The listing builds one solid part. Answer for the finished solid, in the listing's coordinates (mm). Round coordinates to 2 decimals unless told otherwise and drop trailing zeros. Loops run counter-clockwise (first coordinate to the right, second up) from the corner with the lowest first, then second, coordinate; pieces in that order, holes last. Notation, with made-up numbers: (30.25, -2) -> (60.25, -2) arc R12 cw to (60.25, 8) -> close; hole circle Ø6 at (47, -3.75). An arc over 180 degrees is marked (long way). Write each question's results on one line, items separated by ' | '. Start each with the question number.
from build123d import *

# Parameters (mm, degrees)
SM_BASE_FLANGE_1_DEPTH = 3
CUT_EXTRUDE_1_DEPTH    = 10
FILLET_1_R             = 5
FILLET_2_R             = 5
SKETCH_3_R             = 2
CUT_EXTRUDE_2_DEPTH    = 10
SKETCH_5_R             = 2
CUT_EXTRUDE_4_DEPTH    = 10
CHAMFER_1_SIZE         = 1.9
SKETCH_6_R             = 2
CUT_EXTRUDE_5_DEPTH    = 10


# Sheet-metal steps are written as plain solids
with BuildPart() as part:
    # Sketch 1 → Базовая кромка1 (new body)
    with BuildSketch(Plane(origin=(0, 0, 0), x_dir=(1, 0, 0), z_dir=(0, 1, 0))):
        with BuildLine():
            Line((-218.547787293, 260.45511066), (-257.115043875, 306.417777248))
            ThreePointArc((-257.115043875, 306.417777248), (0, 400), (257.115043875, 306.417777248))
            Line((257.115043875, 306.417777248), (218.547787293, 260.45511066))
            ThreePointArc((218.547787293, 260.45511066), (0, 340), (-218.547787293, 260.45511066))
        make_face()
    extrude(amount=-SM_BASE_FLANGE_1_DEPTH)

    # Эскиз2 → Вырез-Вытянуть1 (cut)
    with BuildSketch(Plane(origin=(0, 0, 0), x_dir=(1, 0, 0), z_dir=(0, 1, 0))):
        Polygon((-185.870849123, 267.003439601), (-232.668944094, 335.207852497), (-262.024399195, 311.215696318), (-219.773904278, 254.720487984), align=None)
    extrude(amount=-CUT_EXTRUDE_1_DEPTH, mode=Mode.SUBTRACT)

    # Скругление1
    fillet_1_edges = [part.edges().sort_by_distance(p)[0] for p in [
        (-194.171567718, -1.5, -279.101061069),
        (-228.118354699, -1.5, -328.575738985),
    ]]
    fillet(fillet_1_edges, radius=FILLET_1_R)

    # Скругление2
    fillet_2_edges = [part.edges().sort_by_distance(p)[0] for p in [
        (257.115043875, -1.5, -306.417777248),
        (218.547787293, -1.5, -260.45511066),
    ]]
    fillet(fillet_2_edges, radius=FILLET_2_R)

    # Эскиз3 → Вырез-Вытянуть2 (cut)
    with BuildSketch(Plane(origin=(0, 0, 0), x_dir=(1, 0, 0), z_dir=(0, 1, 0))):
        with Locations(Location((-221.164496487, 327.278574755, 0), (0, 0, 270))):
            Circle(SKETCH_3_R)
        with Locations(Location((-192.875196767, 286.049223862, 0), (0, 0, 270))):
            Circle(SKETCH_3_R)
        with Locations(Location((217.908212497, 267.471514233, 0), (0, 0, 270))):
            Circle(SKETCH_3_R)
        with Locations(Location((250.050541416, 305.777250197, 0), (0, 0, 270))):
            Circle(SKETCH_3_R)
    extrude(amount=-CUT_EXTRUDE_2_DEPTH, mode=Mode.SUBTRACT)

    # Эскиз5 → Вырез-Вытянуть4 (cut)
    with BuildSketch(Plane(origin=(0, 0, 0), x_dir=(1, 0, 0), z_dir=(0, 1, 0))):
        with Locations(Location((15.5203425, 344.65072025, 0), (0, 0, 270))):
            Circle(SKETCH_5_R)
        with Locations(Location((17.7696675, 394.600099996, 0), (0, 0, 270))):
            Circle(SKETCH_5_R)
        with Locations(Location((-106.904799365, 380.258285738, 0), (0, 0, 270))):
            Circle(SKETCH_5_R)
        with Locations(Location((-93.372546281, 332.124325518, 0), (0, 0, 270))):
            Circle(SKETCH_5_R)
    extrude(amount=-CUT_EXTRUDE_4_DEPTH, mode=Mode.SUBTRACT)

    # Фаска1
    chamfer_1_edges = [part.edges().sort_by_distance(p)[0] for p in [
        (-93.372546281, -3, -334.124325518),
        (-221.164496487, -3, -329.278574755),
        (-192.875196767, -3, -288.049223862),
        (217.908212497, -3, -269.471514233),
        (250.050541416, -3, -307.777250197),
        (15.5203425, -3, -346.65072025),
        (17.7696675, -3, -396.600099996),
        (-106.904799365, -3, -382.258285738),
    ]]
    chamfer(chamfer_1_edges, length=CHAMFER_1_SIZE)

    # Эскиз6 → Вырез-Вытянуть5 (cut)
    with BuildSketch(Plane(origin=(0, 0, 0), x_dir=(1, 0, 0), z_dir=(0, 1, 0))):
        with Locations(Location((140.650436017, 369.110355921, 0), (0, 0, 270))):
            Circle(SKETCH_6_R)
        with Locations(Location((122.846583356, 322.387526058, 0), (0, 0, 270))):
            Circle(SKETCH_6_R)
    extrude(amount=-CUT_EXTRUDE_5_DEPTH, mode=Mode.SUBTRACT)


solid = part.part
Item 1: Straight lines are drawn through the part: L1, parallel to X at y = -2.75, z = -296.5; L2, parallel to Z at x = 5.5, y = -0.5; L3, parallel to X at y = -0.65, z = -303. For each, find the intervals that lie inside material, in ascending order. Write a range as [from, to].
Item 2: The part is cut by section C-C, the plane z = -353. Give the vertices of the cut face in (x, y).
Item 3: Determine the mould class of faces 1 (the cylindrical face through (18.4, -1.5, -339.5)), 2 (the flat face through (238.035, -1.479, -283.679)), 3 (the flat face through (18, -3, -363)) for opening direction X: +X half, -X half, draft (parallel to the pull), parting line (faces both ways), or undercut.
Item 4: The part is cut by section A-A, the plane y = -0.6. Give the number of separate pieces and of enclosed holes in the cut face, plus the area to 3 significant figures.
Item 5: Each of these flat-tipped pins is pushed along its axis until it touches: pin 1 Ø3 at (x, z) = (250.05, -305.78) entering from -Y; pin 2 Ø1.5 at (x, y) = (60, -0.5) entering from +Z; pin 3 Ø6.5 at (x, z) = (-192.88, -286.05) entering from -Y; pin 4 Ø1 at (x, y) = (205, -1.5) entering from +Z. Where does it stop, or does it pass through?
Item 6: The part is cut by section B-B, the plane x = 180. Give the vertices of the cut face in (y, z), plus the area to 3 significant figures.
Report:
1) L1: x = [-206.11, -166.4], [166.4, 248.79] | L2: z = [-399.96, -339.96] | L3: x = [-210.57, -154.24], [154.24, 254.21]
2) outline: (-188.12, -3) -> (188.12, -3) -> (188.12, 0) -> (-188.12, 0) -> close
3) face 1: undercut | face 2: +X half | face 3: draft
4) separate pieces: 1 | enclosed holes: 10 | area: 28,800 mm2
5) pin 1: passes through | pin 2: stops at z = -334.53 | pin 3: stops at y = -2.35 | pin 4: stops at z = -270.87
6) outline: (-3, -357.21) -> (0, -357.21) -> (0, -288.44) -> (-3, -288.44) -> close | area: 206 mm2
